from build123d import *

# Parameters (mm, degrees)
F0_W     = 25.4
F0_H     = 25.4
F0_W_2   = 19.05
F0_H_2   = 19.05
F1_DEPTH = 342.9
F3_DEPTH = 25.4


with BuildPart() as f1:
    # F0 (on Top) → F1 (new body)
    with BuildSketch(Plane.XY):
        with Locations((-12.7, 12.7)):
            Rectangle(F0_W, F0_H)
        with Locations((-12.7, 12.7)):
            Rectangle(F0_W_2, F0_H_2, mode=Mode.SUBTRACT)
    extrude(amount=F1_DEPTH)

    # F2 (on face) → F3 (cut)
    with BuildSketch(Plane.YZ):
        Polygon((25.4, 342.9), (0, 342.9), (25.4, 298.905909), align=None)
        Polygon((25.4, 14.664697), (0, 0), (25.4, 0), align=None)
    extrude(amount=-F3_DEPTH, mode=Mode.SUBTRACT)


solid = f1.part
Can you work these out from the model? Positions are in its coordinate system, mm. A direction names the side the tool comes from. Give positions to 0.01 mm unless a question says otherwise; leave off trailing zeros. Write each loop counter-clockwise with the first axis right and the second up, starting at its lowest first coordinate (ties: lowest second). Pieces come first, ordered by that corner, then holes. Notation, with made-up numbers: M 69.25,-19 L 74.25,-19 A20 ccw 74.25,-13 Z; hole C -8,31 d9. An arc over 180 degrees is marked long. Answer in a Markdown table with one row per item. Add a question column.
Item 1: For pin 1 Ø10 at (x, y) = (-21, 19) entering from -Z, with a flat end and sliding along its axis, tell me the tip position at first contact or that it passes through.
Item 2: Imagine slicing it at A-A, the plane y = 13.75. Write out the boundary of the cut face in (x, z) (3 decimals), plus the area to 3 significant figures.
Item 3: Imagine slicing it at C-C, the plane z = 112. Write out the boundary of the cut face in (x, y) (3 decimals), plus the area to 3 significant figures.
Item 4: We'd pull the mould along X, two halves only. Please class faces 1 (the flat face through (0, 13, 169)), 2 (the flat face through (-23.811, 12.878, 7.435)), 3 (the flat face through (-13, 22.225, 157)): released by +X, released by -X, zero draft, split by the parting line, or undercut.
Item 5: Imagine slicing it at B-B, the plane x = -7. Write out the boundary of the cut face in (y, z) (3 decimals).
Item 6: Please list where these lines run through material, in increasing order: L1, parallel to X at y = 11.25, z = 148.5 (3 decimals); L2, parallel to Y at x = -17, z = 240 (3 decimals); L3, parallel to Y at x = -6.75, z = 311.5 (3 decimals).
Item 7: On a 3-axis mill with a long thin cutter (end or side, diameter ignored), from which of +Z, -Z, +X, -X, +Y, -Y can I reach the whole of each face in a straight line? I mean faces 4 (the flat face through (-13, 3.175, 167)), 5 (the flat face through (-23.811, 12.522, 321.211)). Say none if no direction works.
Evaluation:
| question | item | result |
|---|---|---|
| 1 | pin 1 | stops at z = 8.17 |
| 2 | outline | M -25.4,7.939 L -22.225,7.939 L -22.225,319.084 L -25.4,319.084 Z; M -3.175,7.939 L 0,7.939 L 0,319.084 L -3.175,319.084 Z |
| 2 | area | 1,980 mm² |
| 3 | outline | M -25.4,0 L 0,0 L 0,25.4 L -25.4,25.4 Z; hole M -22.225,3.175 L -3.175,3.175 L -3.175,22.225 L -22.225,22.225 Z |
| 3 | area | 282 mm² |
| 4 | face 1 | released by +X |
| 4 | face 2 | zero draft |
| 4 | face 3 | undercut |
| 5 | outline | M 0,0 L 3.175,1.833 L 3.175,337.401 L 0,342.9 Z; M 22.225,12.832 L 25.4,14.665 L 25.4,298.906 L 22.225,304.405 Z |
| 6 | L1 | x = -25.4 to -22.225, -3.175 to 0 |
| 6 | L2 | y = 0 to 3.175, 22.225 to 25.4 |
| 6 | L3 | y = 0 to 3.175 |
| 7 | face 4 | +Z, -Z |
| 7 | face 5 | +Z, +X, -X, +Y |
